Input: part model. Units: mm. Frame: model coordinates. Face numbers are marked on the shaded views. A direction names the side the tool comes from. Coordinates: 2 decimals unless noted, no trailing zeros. Write each loop counter-clockwise with the first axis right and the second up, starting at its lowest first coordinate (ties: lowest second). Pieces come first, ordered by that corner, then holes. Notation, with made-up numbers: (33.25, -36.5) - (37.25, -36.5) arc R35 ccw to (37.25, -3.5) - close; hole circle Ø8 at (24.5, 5). An arc over 180 degrees is marked (long way). One line per question, with ' | ' between items. Start each with the question number.
1) Reachability of the marked faces 1 and 2 from +Z, -Z, +X, -X, +Y, -Y: full face, straight path, thin tool, end or side. Return the list, or none.
2) Section query B-B on z = -17. Return loops of the section in (x, y), and give its area (3 significant figures).
3) Section query A-A on x = 0. Return loops of the section in (y, z).
4) Line query: line 1 (Y direction, x = -22.5, z = -42). Output: solid intervals per line, ascending.
5) First-contact query: P1, Ø2, axis at x = 27, z = -9, coming from the -Y side; P2, Ø8, axis at y = -8.5, z = -30.5, coming from the +X side; P3, Ø22.5, axis at x = 11, y = -26, coming from the -Z side; P4, Ø0.8, axis at y = -12, z = -1, coming from the -X side. Flat tips, straight axial feed; report the tip coordinate or a pass-through.
6) Section query C-C on y = -20. Return loops of the section in (x, z), and give its area (3 significant figures).
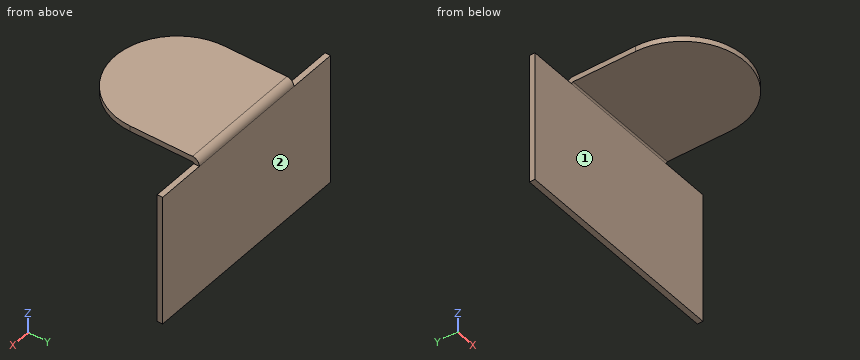
Autodesk Inventor part; units mm, degrees
ref_plane "Work Plane1" through (0, -25, -17) normal (0, 0, 1) x (1, 0, 0)
ref_plane "YZ Plane" through (0, 0, 0) normal (1, 0, 0) x (0, 1, 0)
ref_plane "XZ Plane" through (0, 0, 0) normal (0, 1, 0) x (-1, 0, 0)
sketch "Sketch2" plane through (0, 0, 0) normal (0, 1, 0) x (-1, 0, 0)
  line L0 (22.5, 0) -> (-22.5, 0)
  line L1 (-22.5, 0) -> (-22.5, -50)
  line L2 (-22.5, -50) -> (22.5, -50)
  line L3 (22.5, -50) -> (22.5, 0)
  point P0 (0, 0)
  point P1 (0, 0)
  dimension "d4" = 50
  dimension "d5" = 45
extrude "Extrusion1" add sketch "Sketch2" against normal blind 2
sketch "Sketch3" plane through (0, 0, 0) normal (0, 0, 1) x (1, 0, 0)
  circle A0 centre (0, -25) radius 15.5
  arc A1 (-22.5, -25) -> (22.5, -25) centre (0, -25) ccw
  point P0 (0, 0)
  point P1 (-15.5, -25)
  point P2 (15.5, -25)
  point P3 (-7.75, -11.5766)
  point P4 (7.75, -38.4234)
  point P5 (-7.75, -38.4234)
  point P6 (7.75, -11.5766)
  dimension "d14" = 31
  dimension "d17" = 360
sketch "Sketch4" plane through (0, 0, 0) normal (0, 1, 0) x (1, 0, 0)
  line L0 (-34.5, 43) -> (34.5, 43) construction
  line L1 (34.5, 43) -> (34.5, 9) construction
  line L2 (34.5, 9) -> (-34.5, 9) construction
  line L3 (-34.5, 9) -> (-34.5, 43) construction
  line L4 (22.5, 50) -> (-22.5, 50) construction
  point P0 (0, 0)
  point P1 (0, 43)
  point P2 (0, 50)
  dimension "d26" = 34
  dimension "d27" = 69
  dimension "d36" = 7
sketch "Sketch6" plane through (0, 0, 0) normal (0, 0, 1) x (1, 0, 0)
  line L0 (0, -23) -> (0, -25) construction
  line L1 (-12.5, -23) -> (-12.5, -25)
  line L2 (12.5, -25) -> (12.5, -23)
  arc A0 (12.5, -23) -> (-12.5, -23) centre (0, -23) ccw
  arc A1 (-12.5, -25) -> (12.5, -25) centre (0, -25) ccw
  arc A2 (-22.5, -25) -> (22.5, -25) centre (0, -25) ccw
  point P0 (0, 0)
  point P1 (0, -24)
  dimension "d45" = 25
  dimension "d46" = 2
sketch "Sketch10" plane through (0, -25, -17) normal (0, 0, 1) x (1, 0, 0)
  arc A0 (-12.5, 0) -> (12.5, 0) centre (0, 0) ccw
  circle A1 centre (0, 0) radius 19
  line L0 (0, 0) -> (0, 23) construction
  line L1 (22.5, 23) -> (-22.5, 23)
  line L2 (-22.5, 0) -> (-22.5, 23)
  line L3 (22.5, 23) -> (22.5, 0)
  arc A2 (-22.5, 0) -> (22.5, 0) centre (0, 0) ccw
  arc A3 (22.5, 23) -> (-22.5, 23) centre (0, 23) ccw construction
  arc A4 (-22.5, 0) -> (22.5, 0) centre (0, 0) ccw
  line L4 (37, 23) -> (-37, 23)
  point P0 (19.5, 23)
  point P1 (-19.5, 23)
  point P2 (0, 11.5)
  dimension "d69" = 38
sketch "Sketch12" plane through (-22.5, -25, -2) normal (-1, 0, 0) x (0, 0, 1)
  line L0 (3, 22.5) -> (3, 0)
  line L1 (3, 11) -> (-20, 11)
  line L2 (-20, 11) -> (-34, 23)
  line L3 (-45, 23) -> (-3.5, 23)
  line L4 (-20, 0) -> (-20, 23)
  line L5 (-15, 23) -> (-15, 0)
  line L6 (0, 22.5) -> (0, 0)
  line L7 (0, 22.5) -> (0, 23)
  line L8 (0, 23) -> (-3.5, 23)
  point P0 (2, 25)
  point P1 (-15, 11)
  point P2 (0, 11)
  dimension "d72" = 12
  dimension "d73" = 14
sketch "Sketch1" plane through (0, 0, 0) normal (0, 0, 1) x (1, 0, 0)
  line L0 (0, 0) -> (0, -25) construction
  line L1 (-22.5, 0) -> (-22.5, -25)
  line L2 (22.5, -25) -> (22.5, 0)
  arc A0 (22.5, 0) -> (-22.5, 0) centre (0, 0) ccw construction
  arc A1 (-22.5, -25) -> (22.5, -25) centre (0, -25) ccw
  circle A2 centre (0, -25) radius 18.5 construction
  line L3 (22.5, 0) -> (-22.5, 0)
  line L4 (22.5, 0) -> (22.5, -2)
  line L5 (22.5, -2) -> (-22.5, -2)
  line L6 (-22.5, -2) -> (-22.5, 0)
  line L7 (-22.5, 0) -> (22.5, 0)
  point P0 (0, -12.5)
  point P1 (0, -6.5)
  dimension "d1" = 37
  dimension "d3" = 6.5
sheet face with bend "Face1" sketch "Sketch1" thickness 2 toward (0, 0, -1) bend radius 0.5 contours L5 L2 A1 L1
bend "Bend1"
sketch "Sketch8" plane through (0, 0, 0) normal (0, 1, 0) x (1, 0, 0)
  line L0 (-40, 2.5) -> (40, 2.5)
  line L1 (40, 2.5) -> (40, 50)
  line L2 (40, 50) -> (-40, 50)
  line L3 (-40, 50) -> (-40, 2.5)
  line L4 (-40, 2.5) -> (40, 50) construction
  line L5 (40, 2.5) -> (-40, 50) construction
  line L6 (22.5, 50) -> (-22.5, 50)
  line L7 (-22.5, 2.5) -> (22.5, 2.5)
  point P0 (0, 0)
  point P1 (0, 26.25)
  point P2 (0, 26.25)
  dimension "d50" = 80
extrude "Extrusion3" add sketch "Sketch8" against normal up to surface (2 mm away)
equation "\"d8\" = Thickness"
equation "\"d10\" = BendReliefWidth"
equation "\"d12\" = MinimumRemnant"
equation "\"d11\" = BendReliefDepth"
equation "\"d13\" = TransitionRadius"
equation "\"BendRadius\" = Thickness"
equation "\"BendReliefWidth\" = Thickness"
equation "\"BendReliefDepth\" = 0.5 * Thickness"
equation "\"CornerReliefSize\" = 4 * Thickness"
equation "\"MinimumRemnant\" = 2 * Thickness"
equation "\"TransitionRadius\" = BendRadius"
equation "\"JacobiRadiusSize\" = BendRadius"
equation "\"GapSize\" = Thickness"
properties part number "12v DC motor mount (3D printed)"
Answer key:
1) face 1: -Z, +X, -X, -Y | face 2: +Z, -Z, +X, -X, +Y
2) outline: (-40, -2) - (40, -2) - (40, 0) - (-40, 0) - close | area: 160 mm²
3) outline: (-47.5, -2) - (-2.5, -2) arc R0.5 cw to (-2, -2.5) - (-2, -50) - (0, -50) - (0, -2.5) arc R2.5 ccw to (-2.5, 0) - (-47.5, 0) - close
4) line 1: -2 to 0
5) P1: y = -2 | P2: through | P3: z = -2 | P4: x = -22.5
6) outline: (-22.5, -2) - (22.5, -2) - (22.5, 0) - (-22.5, 0) - close | area: 90.0 mm²
